```python
from build123d import *

# Parameters (mm, degrees)
SKETCH1_R           = 3.175
BOSS_EXTRUDE1_DEPTH = 3.175


with BuildPart() as part:
    # Sketch1 → Boss-Extrude1 (new, symmetric)
    with BuildSketch(Plane(origin=(0, 0, 0), x_dir=(1, 0, 0), z_dir=(0, 1, 0))):
        with BuildLine():
            Line((0, -15.875), (59.24630657, -15.875))
            Line((59.24630657, -15.875), (73.603547963, -19.722011237))
            ThreePointArc((73.603547963, -19.722011237), (75.548098437, -9.946095847), (76.2, 0))
            add(Edge.make_bspline(
                [(76.2, 0), (76.2, 15.875), (0, 15.875)],
                knots=[3.141592654, 3.141592654, 3.141592654, 4.71238898, 4.71238898, 4.71238898], degree=2, weights=[1, 0.707106781, 1]))
            Line((0, 15.875), (-59.24630657, 15.875))
            Line((-59.24630657, 15.875), (-73.603547963, 19.722011237))
            ThreePointArc((-73.603547963, 19.722011237), (-75.548098437, 9.946095847), (-76.2, 0))
            add(Edge.make_bspline(
                [(-76.2, 0), (-76.2, -15.875), (0, -15.875)],
                knots=[3.141592654, 3.141592654, 3.141592654, 4.71238898, 4.71238898, 4.71238898], degree=2, weights=[1, 0.707106781, 1]))
        make_face()
        with Locations(Location((0, 0, 0), (0, 0, 270))):
            Circle(SKETCH1_R, mode=Mode.SUBTRACT)
    extrude(amount=BOSS_EXTRUDE1_DEPTH, both=True)


solid = part.part
```
Geometry: final body of the model. Coordinates: model frame, mm. A direction names the side the tool comes from. Round coordinates to 2 decimals unless told otherwise and drop trailing zeros. Use one line per item in the form item = value. Start each with the question number.
Q1. Access query for faces 4 (the face through (-29, 0, -15.875)), 5 (the face through (29, 0, 15.875)), 6 (the face through (-75.53, 0.04, -10.08)). Directions: +Z, -Z, +X, -X, +Y, -Y. A direction counts if a zero-diameter tool reaches every point of the face in a straight line with its end or side. Return the directions, or none.
Q2. Material intervals for line 1 (X direction, y = -2, z = -2.5); line 2 (X direction, y = -1.25, z = 0.5); line 3 (Z direction, x = 18.5, y = -0.25) (3 decimals), sorted ascending. Write a range as [from, to].
Q3. Pin query (flat end, axial travel): pin 1 Ø3 at (y, z) = (2, 7.5) entering from +X; pin 2 Ø1.5 at (x, y) = (-55.5, 0) entering from +Z; pin 3 Ø3 at (x, y) = (-3.5, -2.5) entering from -Z (3 decimals). Return the tip coordinate at first contact, or that it passes through.
Q4. Mould query, pull axis X, two halves, no side actions, for faces 1 (the face through (75.53, 0.04, 10.08)), 2 (the face through (-1.93, -0.04, -2.52)), 3 (the face through (-1, 3.175, -5)). Classes: +X half, -X half, draft (parallel to the pull), parting line (faces both ways), or undercut.
Geometry results:
q1.face_4 = -Z, +X, +Y, -Y
q1.face_5 = +Z, -X, +Y, -Y
q1.face_6 = -Z, -X, +Y, -Y
q2.line_1 = [-76.16, -1.96], [1.96, 75.25]
q2.line_2 = [-76.16, -3.14], [3.14, 76.2]
q2.line_3 = [-15.4, 15.875]
q3.pin_1 = 75.96
q3.pin_2 = 11.04
q3.pin_3 = -15.875
q4.face_1 = +X half
q4.face_2 = undercut
q4.face_3 = draft
